```python
from build123d import *

# Parameters (mm, degrees)
SKETCH1_R           = 2.425
SKETCH1_R_2         = 1.5
BOSS_EXTRUDE1_DEPTH = 8
BOSS_EXTRUDE2_START = -8
BOSS_EXTRUDE2_DEPTH = 8
CIRPATTERN1_COUNT   = 4
BOSS_EXTRUDE3_DEPTH = 1.25
FILLET1_R           = 0.1


with BuildPart() as part:
    # Sketch1 → Boss-Extrude1 (new body)
    with BuildSketch(Plane(origin=(0, 0, 0), x_dir=(1, 0, 0), z_dir=(0, 1, 0))):
        with Locations(Location((0, 0, 0), (0, 0, 270))):
            Circle(SKETCH1_R)
        with Locations(Location((0, 0, 0), (0, 0, 270))):
            Circle(SKETCH1_R_2, mode=Mode.SUBTRACT)
    extrude(amount=BOSS_EXTRUDE1_DEPTH)

    # Sketch2 → Boss-Extrude2 (add)
    with BuildSketch(Plane(origin=(0, 8, 0), x_dir=(1, 0, 0), z_dir=(0, 1, 0)).offset(BOSS_EXTRUDE2_START)):
        with BuildLine():
            Line((-3.71, -1), (-3.71, 1))
            Line((-3.71, 1), (-2.209213661, 1))
            ThreePointArc((-2.209213661, 1), (-2.425, 0), (-2.209213661, -1))
            Line((-2.209213661, -1), (-3.71, -1))
        make_face()
    boss_extrude2 = extrude(amount=BOSS_EXTRUDE2_DEPTH)

    # CirPattern1: Boss-Extrude2 ×4 about axis
    cirpattern1_axis = Axis((0, 0, 0), (0, 1, 0))
    for i in range(1, CIRPATTERN1_COUNT):
        add(boss_extrude2.rotate(cirpattern1_axis, i * 360 / CIRPATTERN1_COUNT))

    # Sketch3 → Boss-Extrude3 (add)
    with BuildSketch(Plane.XZ):
        with BuildLine():
            Line((-0.538516481, -1.4), (0.538516481, -1.4))
            ThreePointArc((0.538516481, -1.4), (0, -1.5), (-0.538516481, -1.4))
        make_face()
    extrude(amount=-BOSS_EXTRUDE3_DEPTH)

    # Fillet1
    fillet1_edges = [part.edges().sort_by_distance(p)[0] for p in [
        (0, 1.25, -1.5),
    ]]
    fillet(fillet1_edges, radius=FILLET1_R - 0.0001)  # a hair under: the kernel refuses the full size


solid = part.part
```
Work out the finished part from the listing and answer in its coordinate system (mm). A direction names the side the tool comes from. Give positions to 0.01 mm unless a question says otherwise; leave off trailing zeros. Write each loop counter-clockwise with the first axis right and the second up, starting at its lowest first coordinate (ties: lowest second). Pieces come first, ordered by that corner, then holes. Notation, with made-up numbers: (-35, 25) -> (-15, 25) arc R23 cw to (-15, 38) -> close; hole circle Ø3 at (9, 5.5). An arc over 180 degrees is marked (long way). Write each question's results on one line, items separated by ' | '.
1. A tool of negligible diameter and unlimited length cuts with its end or side. For faces 4 (the flat face through (3, 4, -1)), 5 (the flat face through (1, 4, 3)), 6 (the flat face through (-1, 4, 3)), from which of +Z, -Z, +X, -X, +Y, -Y can it reach the whole face along a straight path? Write none if from no direction.
Data:
face 4: -Z, +X, +Y, -Y | face 5: +Z, +X, +Y, -Y | face 6: +Z, -X, +Y, -Y
2. Find section B-B on y = 3.5. Determine the outline of the cut face in (x, z) (3 decimals).
Data:
outline: (-3.71, -1) -> (-2.209, -1) arc R2.425 ccw to (-1, -2.209) -> (-1, -3.71) -> (1, -3.71) -> (1, -2.209) arc R2.425 ccw to (2.209, -1) -> (3.71, -1) -> (3.71, 1) -> (2.209, 1) arc R2.425 ccw to (1, 2.209) -> (1, 3.71) -> (-1, 3.71) -> (-1, 2.209) arc R2.425 ccw to (-2.209, 1) -> (-3.71, 1) -> close; hole circle Ø3 at (0, 0)
3. Determine the mould class of faces 1 (the flat face through (0, 1, -1.4)), 2 (the flat face through (-3, 4, -1)), 3 (the flat face through (1, 4, -3)) for opening direction Z: +Z half, -Z half, draft (parallel to the pull), parting line (faces both ways), or undercut.
Data:
face 1: undercut | face 2: -Z half | face 3: draft
4. Straight lines are drawn through the part: L1, parallel to Z at x = 0, y = 4; L2, parallel to X at y = 2.75, z = 3.25. For each, find the intervals that lie inside material, in ascending order.
Data:
L1: -3.71 to -1.5, 1.5 to 3.71 | L2: -1 to 1
5. Find section C-C on x = 2.75. Determine the outline of the cut face in (y, z).
Data:
outline: (0, -1) -> (8, -1) -> (8, 1) -> (0, 1) -> close
6. Find section D-D on z = 2.5. Determine the outline of the cut face in (x, y).
Data:
outline: (-1, 0) -> (1, 0) -> (1, 8) -> (-1, 8) -> close
7. Find section A-A on z = 0. Determine the outline of the cut face in (x, y).
Data:
outline: (-3.71, 0) -> (-1.5, 0) -> (-1.5, 8) -> (-3.71, 8) -> close; (1.5, 0) -> (3.71, 0) -> (3.71, 8) -> (1.5, 8) -> close
8. Each of these flat-tipped pins is pushed along its axis until it touches: pin 1 Ø1.2 at (x, y) = (3, 4.5) entering from +Z; pin 2 Ø0.8 at (y, z) = (2, -3) entering from -X; pin 3 Ø1.2 at (y, z) = (6, 2.5) entering from +X; pin 4 Ø1 at (x, z) = (-2, -1.5) entering from +Y. Where does it stop, or does it pass through?
Data:
pin 1: z = 1 | pin 2: x = -1 | pin 3: x = 1.51 | pin 4: y = 8
